```python
from build123d import *

# Parameters (mm, degrees)
SKETCH1_W           = 54
SKETCH1_H           = 41
BOSS_EXTRUDE1_DEPTH = 1.5
SKETCH2_W           = 8.89
SKETCH2_H           = 13
BOSS_EXTRUDE2_DEPTH = 8
FILLET1_R           = 2
SKETCH3_W           = 13.765008066
SKETCH3_H           = 5.90131675
BOSS_EXTRUDE3_DEPTH = 5
SKETCH4_R           = 1.5875
CUT_EXTRUDE1_DEPTH  = 10


with BuildPart() as part:
    # Sketch1 → Boss-Extrude1 (new body)
    with BuildSketch(Plane(origin=(0, 0, 0), x_dir=(1, 0, 0), z_dir=(0, 1, 0))):
        with Locations((27, 20.5)):
            Rectangle(SKETCH1_W, SKETCH1_H)
    extrude(amount=BOSS_EXTRUDE1_DEPTH)

    # Sketch2 → Boss-Extrude2 (add)
    with BuildSketch(Plane(origin=(0, 1.5, 0), x_dir=(1, 0, 0), z_dir=(0, 1, 0))):
        with Locations((14.445, 36.5)):
            Rectangle(SKETCH2_W, SKETCH2_H)
    extrude(amount=BOSS_EXTRUDE2_DEPTH)

    # Fillet1
    fillet1_edges = [part.edges().sort_by_distance(p)[0] for p in [
        (0, 0.75, -41),
        (54, 0.75, -41),
        (54, 0.75, 0),
        (0, 0.75, 0),
    ]]
    fillet(fillet1_edges, radius=FILLET1_R)

    # Sketch3 → Boss-Extrude3 (add)
    with BuildSketch(Plane(origin=(0, 1.5, 0), x_dir=(1, 0, 0), z_dir=(0, 1, 0))):
        with Locations((6.882504033, 16.286215299)):
            Rectangle(SKETCH3_W, SKETCH3_H)
    extrude(amount=BOSS_EXTRUDE3_DEPTH)

    # Sketch4 → Cut-Extrude1 (cut)
    with BuildSketch(Plane.ZY):
        with Locations((-16.286215299, 4)):
            Circle(SKETCH4_R)
    extrude(amount=-CUT_EXTRUDE1_DEPTH, mode=Mode.SUBTRACT)


solid = part.part
```
Design review of the part built by this model. Coordinates are the model's own, in mm. A direction names the side the tool comes from. Coordinates: 2 decimals unless noted, no trailing zeros. Order: outer loops, then holes, each group sorted by start corner. A loop starts at its lowest first (then second) coordinate and runs counter-clockwise, first axis right, second up. Notation, with made-up numbers: (-4.5, 72) -> (47.5, 72) arc R14 ccw to (47.5, 87) -> close; hole circle Ø11 at (19, -22). An arc over 180 degrees is marked (long way). One line per item, written item: value. Start each with the question number.
Q1. Insertion check: pin 1 Ø1.5 at (y, z) = (3.5, -36.5) entering from +X; pin 2 Ø2 at (x, y) = (10.5, 5.5) entering from +Z; pin 3 Ø8 at (x, z) = (43, -17) entering from +Y. Each pin has a flat end and moves straight along its axis. Give the tip position at first contact, or say it passes through.
Q2. For probe 1 along X at (y, z) = (2.75, -17) (3 decimals); probe 2 along Y at (x, z) = (52, -40); probe 3 along X at (y, z) = (7, -39), list the stretches that pass through material, from the lowest coordinate up.
Q3. Take a section at C-C, the plane z = -35. State the section outline as (x, y) points, then the cut area to 3 significant figures.
Q4. Take a section at B-B, the plane x = 5. State the section outline as (y, z) points (1 decimal), then the cut area to 3 significant figures.
Q5. Mouldability with a two-part tool opening along Z and no side actions: class faces 6 (the flat face through (27, 1, -41)), 7 (the flat face through (18.89, 5, -36)), 8 (the cylindrical face through (4.93, 3.39, -14.82)) as pulls with the +Z half, pulls with the -Z half, needs draft (parallel to the pull), parting line crosses it, or undercut.
Q6. Take a section at A-A, the plane y = 4. State the section outline as (x, z) points (3 decimals).
Q7. Tool access review of faces 1 (the flat face through (14, 1.5, -42)), 2 (the flat face through (10, 4, -16)), 3 (the flat face through (10, 5, -36)), 4 (the flat face through (7, 4, -19.237)), 5 (the flat face through (7, 6.5, -16)): name each direction out of +Z, -Z, +X, -X, +Y, -Y from which nothing blocks a thin tool from reaching the whole face with its end or side.
Q8. Take a section at D-D, the plane z = -8. State the section outline as (x, y) points, then the cut area to 3 significant figures.
Values follow:
1. pin 1: stops at x = 18.89
1. pin 2: stops at z = -13.34
1. pin 3: stops at y = 1.5
2. probe 1: x = 10 to 13.765
2. probe 2: y = 0 to 1.5
2. probe 3: x = 10 to 18.89
3. outline: (0, 0) -> (54, 0) -> (54, 1.5) -> (18.89, 1.5) -> (18.89, 9.5) -> (10, 9.5) -> (10, 1.5) -> (0, 1.5) -> close
3. area: 152 mm2
4. outline: (0, -41) -> (1.5, -41) -> (1.5, -19.2) -> (6.5, -19.2) -> (6.5, -13.3) -> (1.5, -13.3) -> (1.5, 0) -> (0, 0) -> close; hole circle Ø3.2 at (4, -16.3)
4. area: 83.1 mm2
5. face 6: pulls with the -Z half
5. face 7: needs draft
5. face 8: undercut
6. outline: (0, -19.237) -> (13.765, -19.237) -> (13.765, -13.336) -> (0, -13.336) -> (0, -14.699) -> (10, -14.699) -> (10, -17.874) -> (0, -17.874) -> close; (10, -43) -> (18.89, -43) -> (18.89, -30) -> (10, -30) -> close
7. face 1: -Z, +X, -X, -Y
7. face 2: -X
7. face 3: -Z, -X, +Y
7. face 4: +X, -X, +Y
7. face 5: +Z, +X, -X, +Y
8. outline: (0, 0) -> (54, 0) -> (54, 1.5) -> (0, 1.5) -> close
8. area: 81.0 mm2
